```python
from build123d import *

# Parameters (mm, degrees)
F0_R     = 3.65
F1_DEPTH = 7
F2_START = -4
F2_DEPTH = 3
F3_START = -4
F3_DEPTH = 8


with BuildPart() as f1:
    # F0 (on Top) → F1 (new body)
    with BuildSketch(Plane.XY):
        Circle(F0_R)
    extrude(amount=-F1_DEPTH)

    # F0 (on Top) → F2 (join)
    with BuildSketch(Plane.XY.offset(F2_START)):
        with BuildLine():
            ThreePointArc((-6.15, -5.65), (-6.0035533906, -6.0035533906), (-5.65, -6.15))
            Line((-5.65, -6.15), (5.65, -6.15))
            ThreePointArc((5.65, -6.15), (6.0035533906, -6.0035533906), (6.15, -5.65))
            Line((6.15, -5.65), (6.15, -3.25))
            Line((6.15, -3.25), (6.15, 3.25))
            Line((6.15, 3.25), (6.15, 5.65))
            ThreePointArc((6.15, 5.65), (6.0035533906, 6.0035533906), (5.65, 6.15))
            Line((5.65, 6.15), (-5.65, 6.15))
            ThreePointArc((-5.65, 6.15), (-6.0035533906, 6.0035533906), (-6.15, 5.65))
            Line((-6.15, 5.65), (-6.15, 3.25))
            Line((-6.15, 3.25), (-6.15, -3.25))
            Line((-6.15, -3.25), (-6.15, -5.65))
        make_face()
        Circle(F0_R, mode=Mode.SUBTRACT)
    extrude(amount=-F2_DEPTH)

    # F0 (on Top) → F3 (join)
    with BuildSketch(Plane.XY.offset(F3_START)):
        with BuildLine():
            ThreePointArc((-6.65, -2.75), (-6.5035533906, -3.1035533906), (-6.15, -3.25))
            Line((-6.15, -3.25), (-6.15, 3.25))
            ThreePointArc((-6.15, 3.25), (-6.5035533906, 3.1035533906), (-6.65, 2.75))
            Line((-6.65, 2.75), (-6.65, 0))
            Line((-6.65, 0), (-6.65, -2.75))
        make_face()
        with BuildLine():
            Line((6.15, 3.25), (6.15, -3.25))
            ThreePointArc((6.15, -3.25), (6.5035533906, -3.1035533906), (6.65, -2.75))
            Line((6.65, -2.75), (6.65, 0))
            Line((6.65, 0), (6.65, 2.75))
            ThreePointArc((6.65, 2.75), (6.5035533906, 3.1035533906), (6.15, 3.25))
        make_face()
    extrude(amount=-F3_DEPTH)


solid = f1.part
```
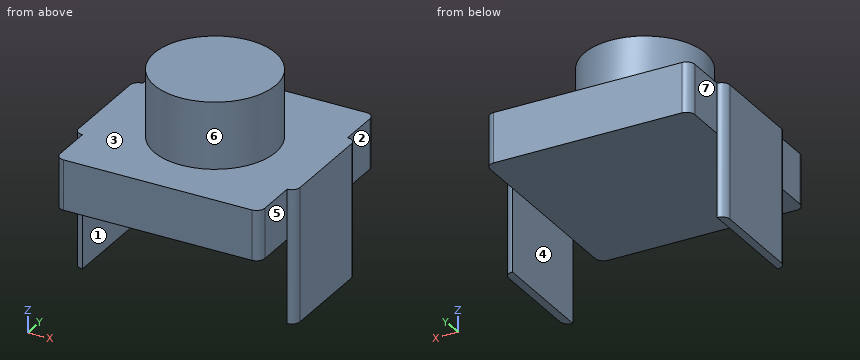
Geometry check sheet. Reference: the model listing, model coordinates, mm. Face numbers are marked on the shaded views. A direction names the side the tool comes from. Give positions to 0.01 mm unless a question says otherwise; leave off trailing zeros. Loops run counter-clockwise (first coordinate to the right, second up) from the corner with the lowest first, then second, coordinate; pieces in that order, holes last. Notation, with made-up numbers: (-11, -13) - (41, -13) arc R10 ccw to (41, -9) - close; hole circle Ø6 at (-17.5, -30.75). An arc over 180 degrees is marked (long way). Use CSV: the item, a comma, the result in double quotes. Start each with the question number.
Q1. Go/stop test with flat-tipped pins: pin 1 Ø1.2 at (y, z) = (-4, -6) entering from +X; pin 2 Ø1 at (x, y) = (1.5, -0.5) entering from -Z; pin 3 Ø2.5 at (y, z) = (-5, -5.5) entering from -X. Record where each tip stops, or that it passes through.
Q2. Access from +Z, -Z, +X, -X, +Y, -Y to the whole of each face (thin tool, end or side, straight path). Record for the marked faces 4, 5, 6 and 7.
Q3. Release check for a two-part mould opening along X. For the marked faces 1, 2 and 3 record: +X half, -X half, draft (parallel to the pull), parting line (faces both ways), or undercut.
Q4. Section check B-B, the plane x = 0. Record the cut outline in (y, z), and give its area (3 significant figures).
Q5. Scan lines: probe 1 along X at (y, z) = (-1.5, -9.25); probe 2 along Z at (x, y) = (-5.5, 3.5); probe 3 along Z at (x, y) = (3.5, 0.75). Record each from-to range of solid material in increasing order. Write a range as from..to.
Q6. Section check D-D, the plane y = 0. Record the cut outline in (x, z), and give its area (3 significant figures).
Q7. Section check A-A, the plane z = -10.5. Record the cut outline in (x, y).
Q8. Section check C-C, the plane z = -6.25. Record the cut outline in (x, y), and give its area (3 significant figures).
Findings below:
1,pin 1,"stops at x = 6.15"
1,pin 2,"stops at z = -7"
1,pin 3,"stops at x = -6.15"
2,face 4,"-Z, +Y, -Y"
2,face 5,"+Z, -Z, +X, -Y"
2,face 6,"+Z"
2,face 7,"+Z, -Z, -X, +Y"
3,face 1,"undercut"
3,face 2,"+X half"
3,face 3,"draft"
4,outline,"(-6.15, -7) - (6.15, -7) - (6.15, -4) - (3.65, -4) - (3.65, 0) - (-3.65, 0) - (-3.65, -4) - (-6.15, -4) - close"
4,area,"66.1 mm^2"
5,probe 1,"x = -6.65..-6.15, 6.15..6.65"
5,probe 2,"z = -7..-4"
5,probe 3,"z = -7..0"
6,outline,"(-6.65, -12) - (-6.15, -12) - (-6.15, -7) - (6.15, -7) - (6.15, -12) - (6.65, -12) - (6.65, -4) - (3.65, -4) - (3.65, 0) - (-3.65, 0) - (-3.65, -4) - (-6.65, -4) - close"
6,area,"74.1 mm^2"
7,outline,"(-6.65, -2.75) arc R0.5 ccw to (-6.15, -3.25) - (-6.15, 3.25) arc R0.5 ccw to (-6.65, 2.75) - close; (6.15, -3.25) arc R0.5 ccw to (6.65, -2.75) - (6.65, 2.75) arc R0.5 ccw to (6.15, 3.25) - close"
8,outline,"(-6.65, -2.75) arc R0.5 ccw to (-6.15, -3.25) - (-6.15, -5.65) arc R0.5 ccw to (-5.65, -6.15) - (5.65, -6.15) arc R0.5 ccw to (6.15, -5.65) - (6.15, -3.25) arc R0.5 ccw to (6.65, -2.75) - (6.65, 2.75) arc R0.5 ccw to (6.15, 3.25) - (6.15, 5.65) arc R0.5 ccw to (5.65, 6.15) - (-5.65, 6.15) arc R0.5 ccw to (-6.15, 5.65) - (-6.15, 3.25) arc R0.5 ccw to (-6.65, 2.75) - close"
8,area,"157 mm^2"
